Answer from the drawing. Dimensions are ordinates in mm from the lowest x, y and z of the part. A direction names the side the tool comes from. Give positions to 0.01 mm unless a question says otherwise; leave off trailing zeros. Loops run counter-clockwise (first coordinate to the right, second up) from the corner with the lowest first, then second, coordinate; pieces in that order, holes last. Notation, with made-up numbers: (53.25, -32.5) - (76.25, -32.5) arc R32 cw to (76.25, 0.5) - close; hole circle Ø3 at (4, 40). An arc over 180 degrees is marked (long way). Answer as CSV lines item,"result". Start each with the question number.
1) For the marked faces 4, 5, 6, 7 and 8, determine the directions among +Z, -Z, +X, -X, +Y, -Y from which every point of the face is accessible in a straight line to the end or side of a thin tool.
2) A cutting plane is placed at A-A (y = 8.25). Determine the outline of the cut face in (x, z).
3) A cutting plane is placed at D-D (y = 16.5). Determine the outline of the cut face in (x, z).
4) A cutting plane is placed at B-B (x = 4.25). Determine the outline of the cut face in (y, z), and give its area (3 significant figures).
5) Find the intervals of material crossed by line 1 along X through (y, z) = (1, 12.25); line 2 along Z through (x, y) = (53.25, 1.35); line 3 along X through (y, z) = (10.5, 12), in increasing order.
6) Flat-ended cylindrical pins translate along their axes: pin 1 (2 mm diameter, centred on x = 54, z = 12.5, fed in from +Y); pin 2 (2.5 mm diameter, centred on x = 5.5, y = 3, fed in from +Z); pin 3 (12 mm diameter, centred on y = 11.5, z = 14, fed in from +X). Find the tip coordinate at first contact, or state that the pin passes through.
7) For a pull along Z with two mould halves and no side action, classify the marked faces 1, 2 and 3 as pulls with the +Z half, pulls with the -Z half, needs draft (parallel to the pull), parting line crosses it, or undercut.
8) A cutting plane is placed at C-C (x = 39.25). Determine the outline of the cut face in (y, z).
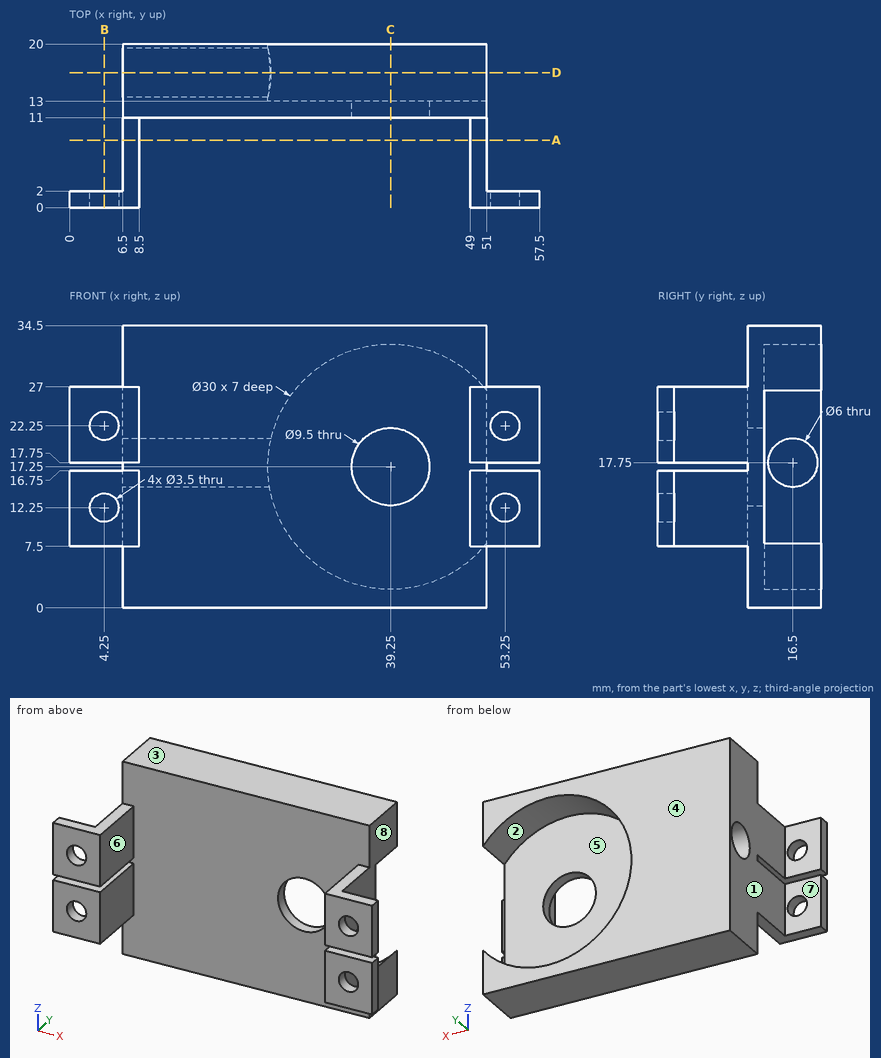
Ans:
1,face 4,"+Z, -Z, +X, -X, +Y"
1,face 5,"+Y"
1,face 6,"+Z, -Z, -Y"
1,face 7,"+Z, -Z, -X, +Y"
1,face 8,"+Z, -Z, +X, +Y"
2,outline,"(6.5, 7.5) - (8.5, 7.5) - (8.5, 16.75) - (6.5, 16.75) - close; (6.5, 17.75) - (8.5, 17.75) - (8.5, 27) - (6.5, 27) - close; (49, 7.5) - (51, 7.5) - (51, 16.75) - (49, 16.75) - close; (49, 17.75) - (51, 17.75) - (51, 27) - (49, 27) - close"
3,outline,"(6.5, 0) - (51, 0) - (51, 7.93) arc R15 cw to (24.46, 14.75) - (6.5, 14.75) - close; (6.5, 20.75) - (24.66, 20.75) arc R15 cw to (51, 26.57) - (51, 34.5) - (6.5, 34.5) - close"
4,outline,"(0, 7.5) - (2, 7.5) - (2, 10.5) - (0, 10.5) - close; (0, 14) - (2, 14) - (2, 16.75) - (0, 16.75) - close; (0, 17.75) - (2, 17.75) - (2, 20.5) - (0, 20.5) - close; (0, 24) - (2, 24) - (2, 27) - (0, 27) - close"
4,area,"23.0 mm2"
5,line 1,"0 to 2.5, 6 to 8.5, 49 to 51.5, 55 to 57.5"
5,line 2,"7.5 to 10.5, 14 to 16.75, 17.75 to 20.5, 24 to 27"
5,line 3,"6.5 to 8.5, 49 to 51"
6,pin 1,"y = 2"
6,pin 2,"z = 27"
6,pin 3,"x = 51"
7,face 1,"needs draft"
7,face 2,"undercut"
7,face 3,"pulls with the +Z half"
8,outline,"(11, 0) - (20, 0) - (20, 2.25) - (13, 2.25) - (13, 12.5) - (11, 12.5) - close; (11, 22) - (13, 22) - (13, 32.25) - (20, 32.25) - (20, 34.5) - (11, 34.5) - close"
